The figure shows three views and two pictorial views of one solid part (mm, origin at its lowest corner). Answer the questions. A direction names the side the tool comes from. Round coordinates to 2 decimals unless told otherwise and drop trailing zeros. Loops run counter-clockwise (first coordinate to the right, second up) from the corner with the lowest first, then second, coordinate; pieces in that order, holes last. Notation, with made-up numbers: (44.25, 0) -> (80.25, 0) arc R21 ccw to (80.25, 31) -> close; hole circle Ø2 at (75, 49.25). An arc over 180 degrees is marked (long way). Write item = value, one per line. Start each with the question number.
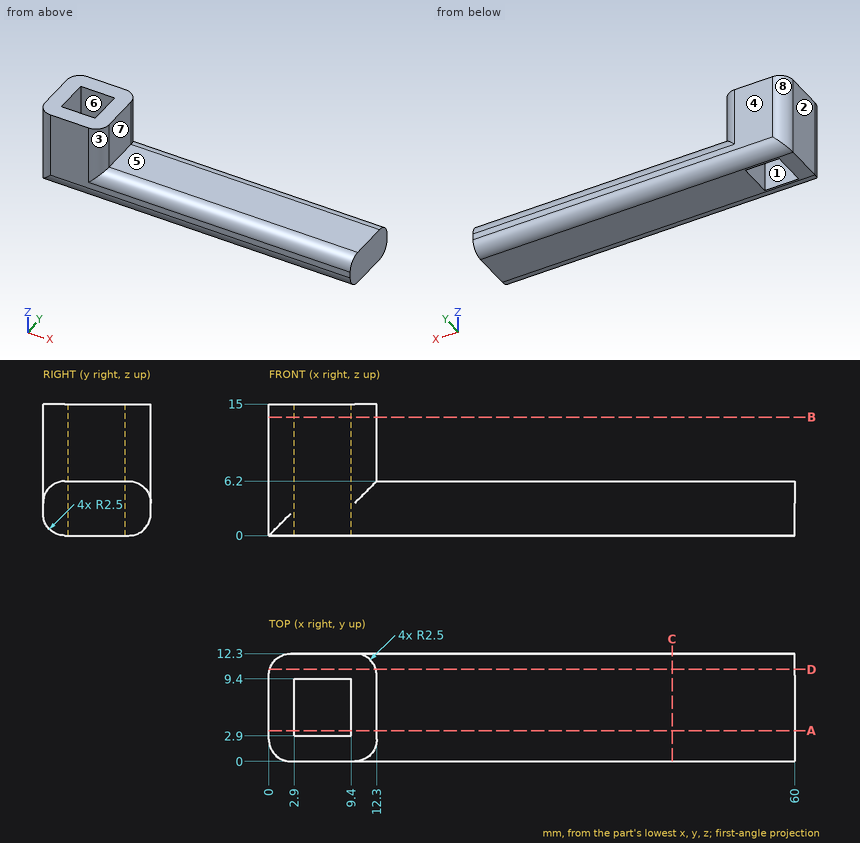
Item 1: Flat-ended cylindrical pins translate along their axes: pin 1 (2 mm diameter, centred on x = 36, y = 6, fed in from +Z); pin 2 (2 mm diameter, centred on y = 7, z = 10, fed in from +X). Find the tip coordinate at first contact, or state that the pin passes through.
Item 2: Section C-C (x = 46) is taken. Determine the outline of the cut face in (y, z), then the cut area to 3 significant figures.
Item 3: A tool of negligible diameter and unlimited length cuts with its end or side. For the marked faces 1, 2, 3, 4 and 5, from which of +Z, -Z, +X, -X, +Y, -Y can it reach the whole face along a straight path? Write none if from no direction.
Item 4: The mould has two halves that part along X. Classify the marked faces 6, 7 and 8: pulls with the +X half, pulls with the -X half, needs draft (parallel to the pull), parting line crosses it, or undercut.
Item 5: Section B-B (z = 13.5) is taken. Determine the outline of the cut face in (x, y).
Item 6: Section D-D (y = 10.5) is taken. Determine the outline of the cut face in (x, z).
Item 7: Section A-A (y = 3.5) is taken. Determine the outline of the cut face in (x, z).
Item 8: Find the intervals of material crossed by line 1 along X through (y, z) = (3.75, 3.5); line 2 along X through (y, z) = (8.5, 11.25), in increasing order. Write a range as [from, to].
Worked answers:
q1.pin_1 = 6.2
q1.pin_2 = 12.3
q2.outline = (0, 2.5) arc R2.5 ccw to (2.5, 0) -> (9.8, 0) arc R2.5 ccw to (12.3, 2.5) -> (12.3, 3.7) arc R2.5 ccw to (9.8, 6.2) -> (2.5, 6.2) arc R2.5 ccw to (0, 3.7) -> close
q2.area = 70.9 mm2
q3.face_1 = +Z, -Z
q3.face_2 = +Z, -Z, -X, +Y, -Y
q3.face_3 = +Z, +X, -Y
q3.face_4 = +Z, -Z, +X, -X, +Y
q3.face_5 = +Z, +X, +Y, -Y
q4.face_6 = undercut
q4.face_7 = pulls with the +X half
q4.face_8 = pulls with the -X half
q5.outline = (0, 2.5) arc R2.5 ccw to (2.5, 0) -> (9.8, 0) arc R2.5 ccw to (12.3, 2.5) -> (12.3, 9.8) arc R2.5 ccw to (9.8, 12.3) -> (2.5, 12.3) arc R2.5 ccw to (0, 9.8) -> close; hole (2.9, 2.9) -> (9.4, 2.9) -> (9.4, 9.4) -> (2.9, 9.4) -> close
q6.outline = (0.1, 0.1) -> (60, 0.1) -> (60, 6.1) -> (12.2, 6.1) -> (12.2, 15) -> (0.1, 15) -> close
q7.outline = (0, 0) -> (2.9, 0) -> (2.9, 15) -> (0, 15) -> close; (9.4, 0) -> (60, 0) -> (60, 6.2) -> (12.3, 6.2) -> (12.3, 15) -> (9.4, 15) -> close
q8.line_1 = [0, 2.9], [9.4, 60]
q8.line_2 = [0, 2.9], [9.4, 12.3]
